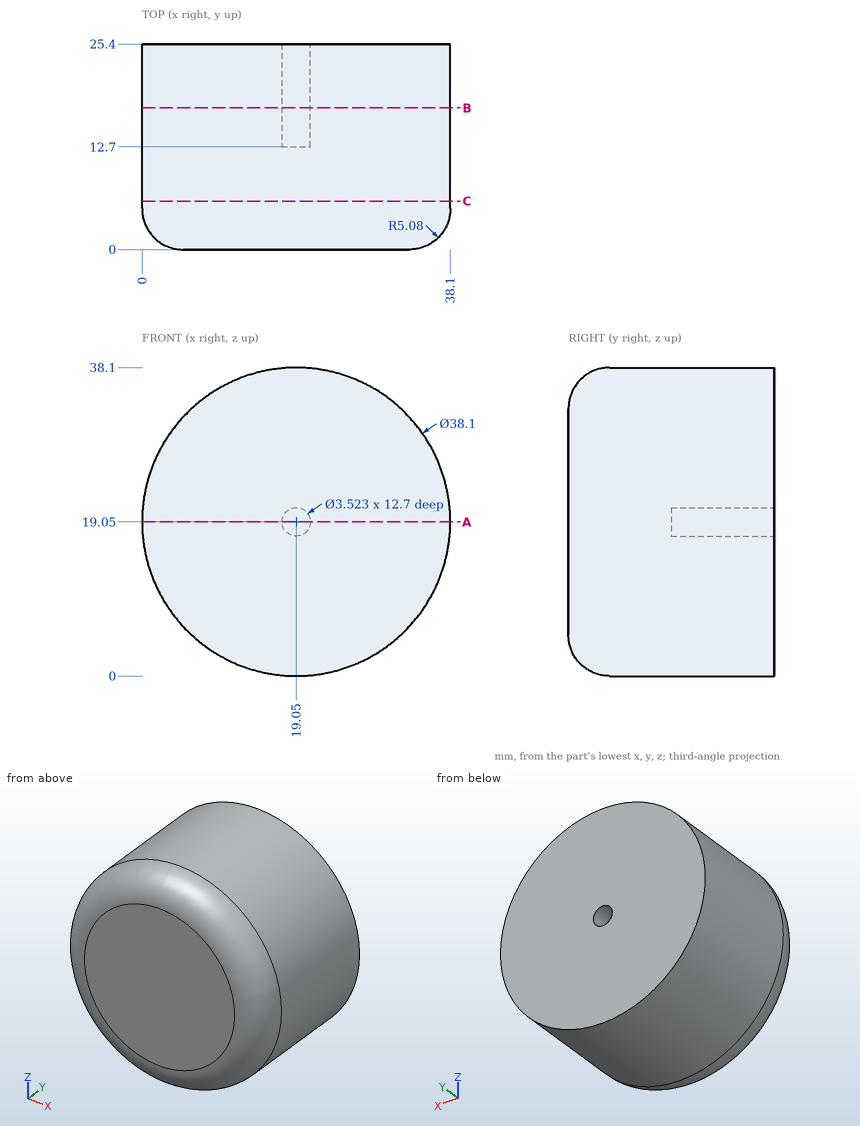
Study the drawing (mm; zero at the part's minimum x, y, z) and answer. Coordinates: 2 decimals unless noted, no trailing zeros. Write each loop counter-clockwise with the first axis right and the second up, starting at its lowest first coordinate (ties: lowest second). Pieces come first, ordered by that corner, then holes.
Q1. A cutting plane is placed at A-A, the plane z = 19.05. Give the vertices of the cut face in (x, y).
Q2. A cutting plane is placed at B-B, the plane y = 17.5. Give the vertices of the cut face in (x, z), then the cut area to 3 significant figures.
Q3. Find the intervals of material crossed by line 1 (Z direction, x = 19.05, y = 22); line 2 (Y direction, x = 19, z = 5), in increasing order.
Q4. A cutting plane is placed at C-C, the plane y = 6. Give the vertices of the cut face in (x, z), then the cut area to 3 significant figures.
Q5. Each of these flat-tipped pins is pushed along its axis until it touches: pin 1 Ø1.5 at (x, z) = (25.5, 33.5) entering from -Y; pin 2 Ø6 at (x, y) = (10.5, 7.5) entering from -Z; pin 3 Ø5 at (x, y) = (27.5, 6) entering from -Z. Where does it stop, or does it pass through?
Findings below:
1. outline: (0, 5.08) arc R5.08 ccw to (5.08, 0) - (33.02, 0) arc R5.08 ccw to (38.1, 5.08) - (38.1, 25.4) - (20.81, 25.4) - (20.81, 12.7) - (17.29, 12.7) - (17.29, 25.4) - (0, 25.4) - close
2. outline: circle Ø38.1 at (19.05, 19.05); hole circle Ø3.52 at (19.05, 19.05)
2. area: 1,130 mm2
3. line 1: z = 0 to 17.29, 20.81 to 38.1
3. line 2: y = 0 to 25.4
4. outline: circle Ø38.1 at (19.05, 19.05)
4. area: 1,140 mm2
5. pin 1: stops at y = 0.12
5. pin 2: stops at z = 0.83
5. pin 3: stops at z = 0.95
